```python
from build123d import *

# Parameters (mm, degrees)
F1_DEPTH = 12
F3_D     = 8
F4_W     = 75
F4_H     = 12
F5_DEPTH = 25


with BuildPart() as f1:
    # F0 (on Front) → F1 (new body)
    with BuildSketch(Plane.XZ):
        with BuildLine():
            Line((332.3978893597, 96.7937542379), (-558.0021106403, 96.7937542379))
            Line((-558.0021106403, 96.7937542379), (-558.0021106403, -4.8062457621))
            Line((-558.0021106403, -4.8062457621), (-436.4021106403, -4.8062457621))
            ThreePointArc((-436.4021106403, -4.8062457621), (-418.7244411107, -12.1285762324), (-411.4021106403, -29.8062457621))
            Line((-411.4021106403, -29.8062457621), (-411.4021106403, -54.8062457621))
            Line((-411.4021106403, -54.8062457621), (-379.4021106403, -54.8062457621))
            Line((-379.4021106403, -54.8062457621), (-379.4021106403, 20.1937542379))
            ThreePointArc((-379.4021106403, 20.1937542379), (-372.07978017, 37.8714237676), (-354.4021106403, 45.1937542379))
            Line((-354.4021106403, 45.1937542379), (-328.4021106403, 45.1937542379))
            ThreePointArc((-328.4021106403, 45.1937542379), (-310.7244411107, 37.8714237676), (-303.4021106403, 20.1937542379))
            Line((-303.4021106403, 20.1937542379), (-303.4021106403, -54.8062457621))
            Line((-303.4021106403, -54.8062457621), (-271.4021106403, -54.8062457621))
            Line((-271.4021106403, -54.8062457621), (-271.4021106403, -29.8062457621))
            ThreePointArc((-271.4021106403, -29.8062457621), (-264.07978017, -12.1285762324), (-246.4021106403, -4.8062457621))
            Line((-246.4021106403, -4.8062457621), (20.7978893597, -4.8062457621))
            ThreePointArc((20.7978893597, -4.8062457621), (38.4755588893, -12.1285762324), (45.7978893597, -29.8062457621))
            Line((45.7978893597, -29.8062457621), (45.7978893597, -54.8062457621))
            Line((45.7978893597, -54.8062457621), (77.7978893597, -54.8062457621))
            Line((77.7978893597, -54.8062457621), (77.7978893597, 20.1937542379))
            ThreePointArc((77.7978893597, 20.1937542379), (85.12021983, 37.8714237676), (102.7978893597, 45.1937542379))
            Line((102.7978893597, 45.1937542379), (128.7978893597, 45.1937542379))
            ThreePointArc((128.7978893597, 45.1937542379), (146.4755588893, 37.8714237676), (153.7978893597, 20.1937542379))
            Line((153.7978893597, 20.1937542379), (153.7978893597, -54.8062457621))
            Line((153.7978893597, -54.8062457621), (185.7978893597, -54.8062457621))
            Line((185.7978893597, -54.8062457621), (185.7978893597, -29.8062457621))
            ThreePointArc((185.7978893597, -29.8062457621), (193.12021983, -12.1285762324), (210.7978893597, -4.8062457621))
            Line((210.7978893597, -4.8062457621), (332.3978893597, -4.8062457621))
            Line((332.3978893597, -4.8062457621), (332.3978893597, 96.7937542379))
        make_face()
    extrude(amount=F1_DEPTH)

    # F3 (through all)
    with Locations(Plane.XZ.offset(12)):
        with Locations((-533.0021106403, 84.0937542379), (-533.0021106403, 58.6937542379), (-533.0021106403, 33.2937542379), (-533.0021106403, 7.8937542379), (331.3978893597, 84.0937542379), (331.3978893597, 58.6937542379), (331.3978893597, 33.2937542379), (331.3978893597, 7.8937542379)):
            Hole(F3_D / 2)

    # F4 (on face) → F5 (cut)
    with BuildSketch(Plane.XZ.offset(12)):
        with Locations((-213.3021106403, 90.7937542379)):
            Rectangle(F4_W, F4_H)
        with Locations((11.6978893597, 90.7937542379)):
            Rectangle(F4_W, F4_H)
    extrude(amount=-F5_DEPTH, mode=Mode.SUBTRACT)


solid = f1.part
```
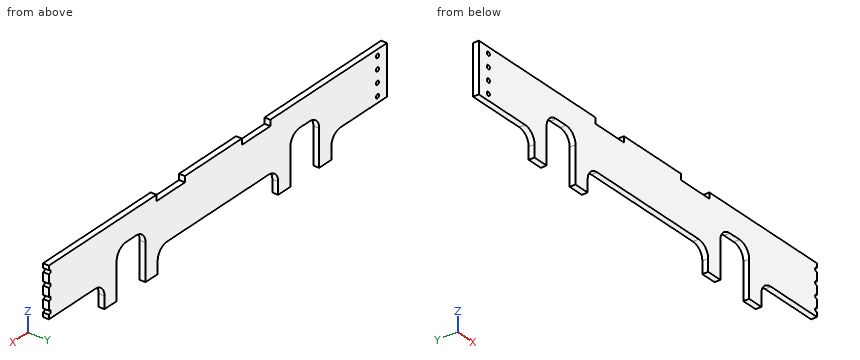
The listing builds one solid part. Answer for the finished solid, in the listing's coordinates (mm). Round coordinates to 2 decimals unless told otherwise and drop trailing zeros. Loops run counter-clockwise (first coordinate to the right, second up) from the corner with the lowest first, then second, coordinate; pieces in that order, holes last. Notation, with made-up numbers: (-38.5, 6) - (-17.5, 6) arc R22 cw to (-17.5, 13) - close; hole circle Ø3 at (89.25, 75). An arc over 180 degrees is marked (long way). Return JSON: item names as keys, results as strings. Group by question number.
1. The part is cut by section D-D on x = -218.5. Determine the outline of the cut face in (y, z), then the cut area to 3 significant figures.
2. Each of these flat-tipped pins is pushed along its axis until it touches: P1, Ø3.5, axis at x = 267, y = -8, coming from the -Z side; P2, Ø6, axis at y = -5.5, z = -32.5, coming from the -X side; P3, Ø4, axis at y = -6.5, z = -11, coming from the -X side. Where does it stop, or does it pass through?
3. Consider probe 1 along X at (y, z) = (-6.25, 21); probe 2 along X at (y, z) = (-9.25, -34.5); probe 3 along X at (y, z) = (-8, -27). Determine where each line is inside the solid, lowest interval first.
4. The part is cut by section A-A on z = -15.5. Determine the outline of the cut face in (x, y), then the cut area to 3 significant figures.
5. The part is cut by section B-B on x = 227. Determine the outline of the cut face in (y, z), then the cut area to 3 significant figures.
6. The part is cut by section C-C on y = -2.5. State how many separate pieces and enclosed holes the cut face has, then the cut area to 3 significant figures.
Resolved:
{
 "1": {"outline": "(-12, -4.81) - (0, -4.81) - (0, 84.79) - (-12, 84.79) - close", "area": "1,080 mm²"},
 "2": {"P1": "stops at z = -4.81", "P2": "stops at x = -411.4", "P3": "stops at x = -422.54"},
 "3": {"probe 1": "x = -558 to -379.39, -303.42 to 77.81, 153.78 to 332.4", "probe 2": "x = -411.4 to -379.4, -303.4 to -271.4, 45.8 to 77.8, 153.8 to 185.8", "probe 3": "x = -411.56 to -379.4, -303.4 to -271.24, 45.64 to 77.8, 153.8 to 185.96"},
 "4": {"outline": "(-415.9, -12) - (-379.4, -12) - (-379.4, 0) - (-415.9, 0) - close; (-303.4, -12) - (-266.9, -12) - (-266.9, 0) - (-303.4, 0) - close; (41.3, -12) - (77.8, -12) - (77.8, 0) - (41.3, 0) - close; (153.8, -12) - (190.3, -12) - (190.3, 0) - (153.8, 0) - close", "area": "1,750 mm²"},
 "5": {"outline": "(-12, -4.81) - (0, -4.81) - (0, 96.79) - (-12, 96.79) - close", "area": "1,220 mm²"},
 "6": {"separate pieces": "1", "enclosed holes": "4", "area": "88,200 mm²"}
}
